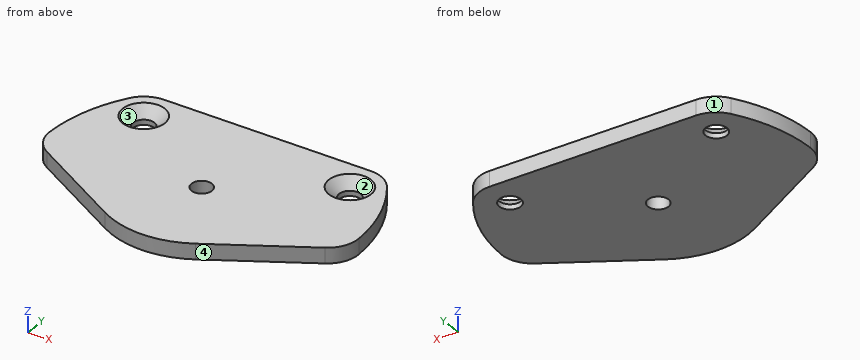
```python
from build123d import *

# Parameters (mm, degrees)
SKETCH_1_R      = 2.1
SKETCH_1_R_2    = 2
EXTRUDE_1_DEPTH = 1.5
CHAMFER_1_SIZE  = 2


with BuildPart() as part:
    # 草图1 → 凸台-拉伸1 (new, symmetric)
    with BuildSketch(Plane.XY):
        with BuildLine():
            Line((-20, 19.266499161), (20, 19.266499161))
            ThreePointArc((20, 19.266499161), (22.837274331, 18.553263235), (25, 16.583123952))
            ThreePointArc((25, 16.583123952), (28.617303042, 9.002775495), (29.991436749, 0.716743841))
            ThreePointArc((29.991436749, 0.716743841), (29.224770759, -2.364314571), (26.993149399, -4.62275735))
            Line((26.993149399, -4.62275735), (8.75, -15.155444566))
            ThreePointArc((8.75, -15.155444566), (0, -17.5), (-8.75, -15.155444566))
            Line((-8.75, -15.155444566), (-26.993149399, -4.62275735))
            ThreePointArc((-26.993149399, -4.62275735), (-29.224770759, -2.364314571), (-29.991436749, 0.716743841))
            ThreePointArc((-29.991436749, 0.716743841), (-28.617303042, 9.002775495), (-25, 16.583123952))
            ThreePointArc((-25, 16.583123952), (-22.837274331, 18.553263235), (-20, 19.266499161))
        make_face()
        with Locations((-20, 13.266499161)):
            Circle(SKETCH_1_R, mode=Mode.SUBTRACT)
        with Locations((20, 13.266499161)):
            Circle(SKETCH_1_R, mode=Mode.SUBTRACT)
        Circle(SKETCH_1_R_2, mode=Mode.SUBTRACT)
    extrude(amount=EXTRUDE_1_DEPTH, both=True)

    # 倒角1
    chamfer_1_edges = [part.edges().sort_by_distance(p)[0] for p in [
        (-22.1, 13.266499161, 1.5),
        (17.9, 13.266499161, 1.5),
    ]]
    chamfer(chamfer_1_edges, length=CHAMFER_1_SIZE)


solid = part.part
```
Source: CAD feature listing. Evaluate the final solid. Frame: model axes, mm. Face numbers are marked on the shaded views. Coordinates: 2 decimals unless noted, no trailing zeros. Loops run counter-clockwise (first coordinate to the right, second up) from the corner with the lowest first, then second, coordinate; pieces in that order, holes last. Notation, with made-up numbers: (-17.75, 7.5) - (2.25, 7.5) arc R7 ccw to (2.25, 20.5) - close; hole circle Ø11 at (88, 30). An arc over 180 degrees is marked (long way). Answer as CSV lines item,"result".
1. Section D-D (x = 15). Return loops of the section in (y, z).
Established:
outline,"(-11.55, -1.5) - (19.27, -1.5) - (19.27, 1.5) - (-11.55, 1.5) - close"
2. Mould query, pull axis Y, two halves, no side actions, for the marked faces 1, 2, 3 and 4. Classes: released by +Y, released by -Y, zero draft, split by the parting line, or undercut.
Established:
face 1,"released by +Y"
face 2,"undercut"
face 3,"undercut"
face 4,"released by -Y"
3. Ray query, line 1 (Y direction, x = 0, z = -0.85); line 2 (X direction, y = 12, z = -0.5); line 3 (X direction, y = 1.5, z = 1). Return the intervals inside material, ascending.
Established:
line 1,"y = -17.5 to -2, 2 to 19.27"
line 2,"x = -27.5 to -21.68, -18.32 to 18.32, 21.68 to 27.5"
line 3,"x = -29.96 to -1.32, 1.32 to 29.96"
4. Section A-A (x = 0). Return loops of the section in (y, z), then the cut area to 3 significant figures.
Established:
outline,"(-17.5, -1.5) - (-2, -1.5) - (-2, 1.5) - (-17.5, 1.5) - close; (2, -1.5) - (19.27, -1.5) - (19.27, 1.5) - (2, 1.5) - close"
area,"98.3 mm2"
5. Section C-C (y = 0). Return loops of the section in (x, z), then the cut area to 3 significant figures.
Established:
outline,"(-29.97, -1.5) - (-2, -1.5) - (-2, 1.5) - (-29.97, 1.5) - close; (2, -1.5) - (29.97, -1.5) - (29.97, 1.5) - (2, 1.5) - close"
area,"168 mm2"
6. Section B-B (z = -1.05). Return loops of the section in (x, y), then the cut area to 3 significant figures.
Established:
outline,"(-29.99, 0.72) arc R6 ccw to (-26.99, -4.62) - (-8.75, -15.16) arc R17.5 ccw to (8.75, -15.16) - (26.99, -4.62) arc R6 ccw to (29.99, 0.72) arc R30 ccw to (25, 16.58) arc R6 ccw to (20, 19.27) - (-20, 19.27) arc R6 ccw to (-25, 16.58) arc R30 ccw to start; hole circle Ø4.2 at (-20, 13.27); hole circle Ø4 at (0, 0); hole circle Ø4.2 at (20, 13.27)"
area,"1,700 mm2"
